Input: part model. Units: mm. Frame: model coordinates. A direction names the side the tool comes from. Coordinates: 2 decimals unless noted, no trailing zeros. Order: outer loops, then holes, each group sorted by start corner. A loop starts at its lowest first (then second) coordinate and runs counter-clockwise, first axis right, second up. Notation, with made-up numbers: (-11.75, -19) -> (45.25, -19) arc R6 ccw to (45.25, -13) -> close; hole circle Ø6 at (60.5, 75.25). An arc over 180 degrees is marked (long way). One line per question, with ' | ' between items.
```python
from build123d import *

# Parameters (mm, degrees)
BOSS_EXTRUDE1_DEPTH = 20
SKETCH3_OUTSIDE_W   = 154.97
SKETCH3_OUTSIDE_H   = 154.97
SKETCH3_OUTSIDE_R   = 22.5
CUT_EXTRUDE1_DEPTH  = 20
CUT_EXTRUDE1_TAPER  = 60
CUT_EXTRUDE2_REACH  = 22
SKETCH4_R           = 15


with BuildPart() as part:
    # Sketch1 → Boss-Extrude1 (new body)
    with BuildSketch(Plane.XY):
        Polygon((0, 25.980762114), (-22.5, 12.990381057), (-22.5, -12.990381057), (0, -25.980762114), (22.5, -12.990381057), (22.5, 12.990381057), align=None)
    extrude(amount=BOSS_EXTRUDE1_DEPTH)

    # Sketch2 → Revolve2 (revolve)
    with BuildSketch(Plane(origin=(0, 0, 0), x_dir=(0, 0, -1), z_dir=(1, 0, 0))):
        with BuildLine():
            Line((0, 0), (-12, 0))
            ThreePointArc((-12, 0), (-9.145772075, -17.058051419), (-0.894027207, -32.257802794))
            ThreePointArc((-0.894027207, -32.257802794), (-0.337232687, -32.42276506), (0, -31.95))
            Line((0, -31.95), (0, 0))
        make_face()
    revolve(axis=Axis((0, 0, 0), (0, 0, 1)))

    # Sketch3 outside → Cut-Extrude1 (cut)
    with BuildSketch(Plane.XY.offset(20)):
        Rectangle(SKETCH3_OUTSIDE_W, SKETCH3_OUTSIDE_H)
        Circle(SKETCH3_OUTSIDE_R, mode=Mode.SUBTRACT)
    extrude(amount=-CUT_EXTRUDE1_DEPTH, taper=CUT_EXTRUDE1_TAPER, mode=Mode.SUBTRACT)

    # Sketch4 → Cut-Extrude2 (cut, up to next)
    with BuildSketch(Plane.XY.offset(20), mode=Mode.PRIVATE) as cut_extrude2_sk1:
        Circle(SKETCH4_R)
    cut_extrude2_tool1 = extrude(cut_extrude2_sk1.sketch, amount=-CUT_EXTRUDE2_REACH, mode=Mode.PRIVATE) & part.part
    add(cut_extrude2_tool1.solids().sort_by_distance((0, 0, 20))[0], mode=Mode.SUBTRACT)


solid = part.part
```
1. Pin query (flat end, axial travel): pin 1 Ø12 at (y, z) = (5.5, 11) entering from +X; pin 2 Ø3 at (x, z) = (4, 3.5) entering from +Y; pin 3 Ø6 at (y, z) = (2, 16) entering from -X. Return the tip coordinate at first contact, or that it passes through.
Recorded:
pin 1: stops at x = 25.65 | pin 2: stops at y = 30.54 | pin 3: stops at x = -22.5
2. Access query for faces 1 (the face through (11.09, -19.58, 12.45)), 2 (the face through (11.4, 19.4, 12.4)), 3 (the face through (-11.4, -19.4, 12.4)). Directions: +Z, -Z, +X, -X, +Y, -Y. A direction counts if a zero-diameter tool reaches every point of the face in a straight line with its end or side. Return the directions, or none.
Recorded:
face 1: +Z, +X, -Y | face 2: +Z, +X, +Y | face 3: +Z, -X, -Y
3. Ray query, line 1 (Y direction, x = 0, z = 6.5); line 2 (Y direction, x = -10.5, z = 3); line 3 (X direction, y = 13, z = 5.75). Return the intervals inside material, ascending. Write a range as [from, to].
Recorded:
line 1: y = [-25.98, -15], [15, 25.98] | line 2: y = [-27.42, -10.71], [10.71, 27.42] | line 3: x = [-22.48, -7.48], [7.48, 22.48]
4. Cut plane A-A, the plane z = 13. Return loops of the section in (x, y), and give its area (3 significant figures).
Recorded:
outline: (-22.5, -12.99) -> (0, -25.98) -> (22.5, -12.99) -> (22.5, 12.99) -> (0, 25.98) -> (-22.5, 12.99) -> close; hole circle Ø30 at (0, 0) | area: 1,050 mm^2
5. Mould query, pull axis X, two halves, no side actions, for faces 4 (the face through (0.06, -23.35, 19.51)), 5 (the face through (-14.985, 0.66, 10.14)), 6 (the face through (-20.19, -11.72, 19.51)). Classes: released by +X, released by -X, zero draft, split by the parting line, or undercut.
Recorded:
face 4: split by the parting line | face 5: undercut | face 6: released by -X
